```python
from build123d import *

# Parameters (mm, degrees)
SKETCH2_R           = 9.271
BOSS_EXTRUDE1_DEPTH = 1.651
SKETCH2_3_R         = 7.874
SKETCH2_3_R_2       = 5.1435
SKETCH2_3_R_3       = 4.826
SKETCH2_3_R_4       = 2.159
SKETCH2_3_R_5       = 1.905
CUT_EXTRUDE1_DEPTH  = 0.0254
SKETCH3_R           = 1.186010715
CUT_EXTRUDE2_DEPTH  = 0.0254


with BuildPart() as part:
    # Sketch2 → Boss-Extrude1 (new body)
    with BuildSketch(Plane(origin=(0, 0, 0), x_dir=(1, 0, 0), z_dir=(0, 1, 0))):
        with Locations(Location((0, 0, 0), (0, 0, 90))):
            Circle(SKETCH2_R)
    extrude(amount=BOSS_EXTRUDE1_DEPTH)

    # Sketch2_3 → Cut-Extrude1 (cut)
    # profile 1 of 3: a face of its own
    with BuildSketch(Plane(origin=(0, 0, 0), x_dir=(1, 0, 0), z_dir=(0, 1, 0))):
        with Locations(Location((0, 0, 0), (0, 0, 270))):
            Circle(SKETCH2_3_R)
        with Locations(Location((0, 0, 0), (0, 0, 270))):
            Circle(SKETCH2_3_R_2, mode=Mode.SUBTRACT)
    # profile 2 of 3: a face of its own
    with BuildSketch(Plane(origin=(0, 0, 0), x_dir=(1, 0, 0), z_dir=(0, 1, 0))):
        with Locations(Location((0, 0, 0), (0, 0, 270))):
            Circle(SKETCH2_3_R_3)
        with Locations(Location((0, 0, 0), (0, 0, 270))):
            Circle(SKETCH2_3_R_4, mode=Mode.SUBTRACT)
    # profile 3 of 3: a face of its own
    with BuildSketch(Plane(origin=(0, 0, 0), x_dir=(1, 0, 0), z_dir=(0, 1, 0))):
        with Locations(Location((0, 0, 0), (0, 0, 270))):
            Circle(SKETCH2_3_R_5)
    extrude(amount=CUT_EXTRUDE1_DEPTH, mode=Mode.SUBTRACT)

    # Sketch3 → Cut-Extrude2 (cut)
    with BuildSketch(Plane(origin=(0, 1.651, 0), x_dir=(1, 0, 0), z_dir=(0, 1, 0))):
        with Locations(Location((-2.88114027, 3.706360639, 0), (0, 0, 270))):
            Circle(SKETCH3_R)
        with Locations(Location((0, 3.706360639, 0), (0, 0, 270))):
            Circle(SKETCH3_R)
        with Locations(Location((2.88114027, 3.706360639, 0), (0, 0, 270))):
            Circle(SKETCH3_R)
        with Locations(Location((0, -3.706360639, 0), (0, 0, 270))):
            Circle(SKETCH3_R)
        with Locations(Location((-2.88114027, -3.706360639, 0), (0, 0, 270))):
            Circle(SKETCH3_R)
        with Locations(Location((2.88114027, -3.706360639, 0), (0, 0, 270))):
            Circle(SKETCH3_R)
    extrude(amount=-CUT_EXTRUDE2_DEPTH, mode=Mode.SUBTRACT)


solid = part.part
```
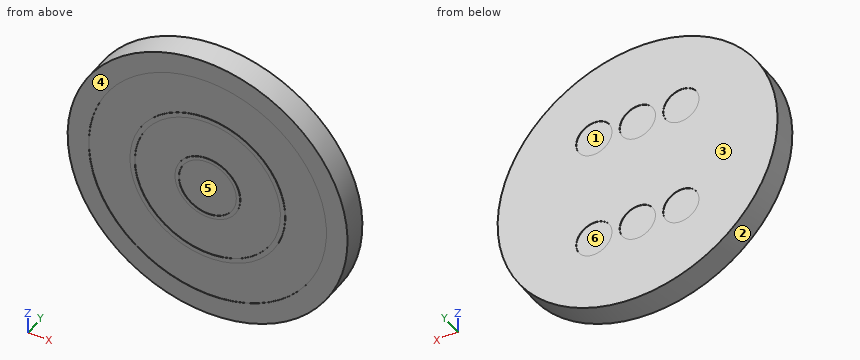
Design review of the part built by this model. Coordinates are the model's own, in mm. Face numbers are marked on the shaded views. A direction names the side the tool comes from. Coordinates: 2 decimals unless noted, no trailing zeros. Loops run counter-clockwise (first coordinate to the right, second up) from the corner with the lowest first, then second, coordinate; pieces in that order, holes last.
Q1. Tool access review of the marked faces 4, 5 and 6: name each direction out of +Z, -Z, +X, -X, +Y, -Y from which nothing blocks a thin tool from reaching the whole face with its end or side.
Reported:
face 4: +Z, -Z, +X, -X, -Y
face 5: -Y
face 6: +Y
Q2. The part is to be moulded in two halves that separate along X. For the marked faces 1, 2 and 3, say which applies: +X half, -X half, draft (parallel to the pull), parting line (faces both ways), or undercut.
Reported:
face 1: undercut
face 2: parting line
face 3: draft
Q3. For pin 1 (1.9 mm diameter, centred on x = 0, z = 3.71, fed in from +Y); pin 2 (1 mm diameter, centred on x = 2, z = -3.5, fed in from -Y), all flat-tipped, find the tip position at first contact; note any pin that passes through.
Reported:
pin 1: stops at y = 1.63
pin 2: stops at y = 0.03
Q4. To check wall thickness, follow line 1 (Y direction, x = 5.5, z = -4.5); line 2 (X direction, y = 1.45, z = 0.25). State the ranges of each line that lie inside material, in increasing order.
Reported:
line 1: y = 0.03 to 1.65
line 2: x = -9.27 to 9.27
Q5. We need section C-C on y = 0.95. State the section outline as (x, z) points.
Reported:
outline: circle Ø18.54 at (0, 0)
